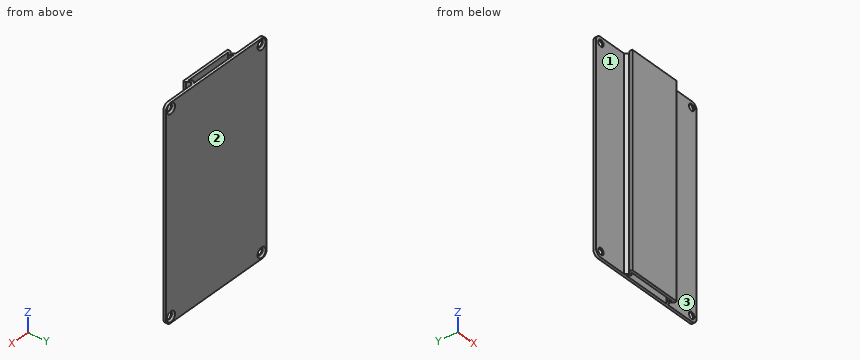
```python
from build123d import *

# Parameters (mm, degrees)
BOSS_EXTRUDE1_DEPTH = 60
CUT_EXTRUDE1_START  = -7.2
SKETCH7_R           = 1.875
CUT_EXTRUDE1_DEPTH  = 8.2
CHAMFER1_SIZE       = 1
FILLET1_R           = 3


with BuildPart() as part:
    # Sketch2 → Boss-Extrude1 (new body, symmetric)
    with BuildSketch(Plane.XY):
        Polygon((0, 0), (-35, 0), (-35, -1.5), (-15.5, -1.5), (-13.9, -3.1), (-15.5, -4.7), (-15.5, -6.2), (0, -6.2), (0, -4.7), (-14, -4.7), (-12.4, -3.1), (-14, -1.5), (0, -1.5), align=None)
    boss_extrude1 = extrude(amount=BOSS_EXTRUDE1_DEPTH, both=True)

    # Sketch7 → Cut-Extrude1 (cut)
    with BuildSketch(Plane(origin=(0, 0, 0), x_dir=(1, 0, 0), z_dir=(0, 1, 0)).offset(CUT_EXTRUDE1_START)):
        with Locations((-31.625, 56.625)):
            Circle(SKETCH7_R)
        with Locations((-31.625, -56.625)):
            Circle(SKETCH7_R)
    cut_extrude1 = extrude(amount=CUT_EXTRUDE1_DEPTH, mode=Mode.SUBTRACT)

    # Mirror1: Boss-Extrude1, Cut-Extrude1 across plane
    add(boss_extrude1.mirror(Plane(origin=(0, -4.7, 60), x_dir=(0, 0, 1), z_dir=(-1, 0, 0))))
    add(cut_extrude1.mirror(Plane(origin=(0, -4.7, 60), x_dir=(0, 0, 1), z_dir=(-1, 0, 0))), mode=Mode.SUBTRACT)

    # Chamfer1
    chamfer1_edges = [part.edges().sort_by_distance(p)[0] for p in [
        (-33.5, 0, -56.625),
        (-33.5, 0, 56.625),
        (33.5, 0, -56.625),
        (33.5, 0, 56.625),
    ]]
    chamfer(chamfer1_edges, length=CHAMFER1_SIZE)

    # Fillet1
    fillet1_edges = [part.edges().sort_by_distance(p)[0] for p in [
        (-35, -0.75, 60),
        (-35, -0.75, -60),
        (35, -0.75, 60),
        (35, -0.75, -60),
    ]]
    fillet(fillet1_edges, radius=FILLET1_R)


solid = part.part
```
Design review of the part built by this model. Coordinates are the model's own, in mm. Face numbers are marked on the shaded views. A direction names the side the tool comes from. Coordinates: 2 decimals unless noted, no trailing zeros. Order: outer loops, then holes, each group sorted by start corner. A loop starts at its lowest first (then second) coordinate and runs counter-clockwise, first axis right, second up. Notation, with made-up numbers: (78.5, 76.25) - (136.5, 76.25) arc R29 cw to (136.5, 102.25) - close; hole circle Ø7 at (55.5, -34). An arc over 180 degrees is marked (long way). Answer in a Markdown table with one row per item.
(1) Clearance check with flat-ended pins moving along their axes: pin 1 (4.5 mm diameter, centred on x = 31.625, z = 56.625, fed in from +Y) (3 decimals); pin 2 (15.5 mm diameter, centred on x = -28, z = 28.5, fed in from -Y); pin 3 (1.6 mm diameter, centred on y = -5, z = -15.5, fed in from +X); pin 4 (2 mm diameter, centred on x = -31.625, z = 56.625, fed in from -Y). State where each tip first meets the part, or that it passes through.
Checked values:
| item | result |
|---|---|
| pin 1 | y = -0.625 |
| pin 2 | y = -1.5 |
| pin 3 | x = 15.5 |
| pin 4 | through |
(2) Consider section A-A on x = -5.5. State the section outline as (y, z) points, plus the area to 3 significant figures.
Checked values:
| item | result |
|---|---|
| outline | (-6.2, -60) - (-4.7, -60) - (-4.7, 60) - (-6.2, 60) - close; (-1.5, -60) - (0, -60) - (0, 60) - (-1.5, 60) - close |
| area | 360 mm^2 |
(3) For the marked faces 1, 2 and 3, list the 3-axis set-ups (+Z, -Z, +X, -X, +Y, -Y) from which the entire face can be reached by the end or side of a thin tool; tool diameter is ignored.
Checked values:
| item | result |
|---|---|
| face 1 | +Z, -Z, -X, -Y |
| face 2 | +Z, -Z, +X, -X, +Y |
| face 3 | +Z, -Z, +X, -Y |
(4) Consider section B-B on z = -5. State the section outline as (x, y) points.
Checked values:
| item | result |
|---|---|
| outline | (-35, -1.5) - (-15.5, -1.5) - (-13.9, -3.1) - (-15.5, -4.7) - (-15.5, -6.2) - (15.5, -6.2) - (15.5, -4.7) - (13.9, -3.1) - (15.5, -1.5) - (35, -1.5) - (35, 0) - (-35, 0) - close; hole (-14, -4.7) - (14, -4.7) - (12.4, -3.1) - (14, -1.5) - (-14, -1.5) - (-12.4, -3.1) - close |
(5) Consider section C-C on x = -24.5. State the section outline as (y, z) points.
Checked values:
| item | result |
|---|---|
| outline | (-1.5, -60) - (0, -60) - (0, 60) - (-1.5, 60) - close |
(6) Wall thickness on line 1 along Y through (x, z) = (12, -33); line 2 along X through (y, z) = (-5.5, -25.5); line 3 along Y through (x, z) = (-24.5, -49.5): over which ranges is each line inside the solid? List them lowest first. Write a range as from..to.
Checked values:
| item | result |
|---|---|
| line 1 | -6.2..-4.7, -1.5..0 |
| line 2 | -15.5..15.5 |
| line 3 | -1.5..0 |
